The listing builds one solid part. Answer for the finished solid, in the listing's coordinates (mm). A direction names the side the tool comes from. Coordinates: 2 decimals unless noted, no trailing zeros. Write each loop counter-clockwise with the first axis right and the second up, starting at its lowest first coordinate (ties: lowest second). Pieces come first, ordered by that corner, then holes.
from build123d import *

# Parameters (mm, degrees)
F0_R     = 14.75
F1_DEPTH = 5
F2_R     = 5.25
F2_R_2   = 2.75
F3_DEPTH = 5
F4_R     = 0.5


with BuildPart() as f1:
    # F0 (on Top) → F1 (new body)
    with BuildSketch(Plane.XY):
        Circle(F0_R)
    extrude(amount=F1_DEPTH)

    # F2 (on face) → F3 (join)
    with BuildSketch(Plane.XY.offset(5)):
        Circle(F2_R)
        Circle(F2_R_2, mode=Mode.SUBTRACT)
    extrude(amount=F3_DEPTH)

    # F4
    f4_edges = [f1.edges().sort_by_distance(p)[0] for p in [
        (-14.75, 0, 0),
        (-2.75, 0, 10),
    ]]
    fillet(f4_edges, radius=F4_R)


solid = f1.part
Q1. Determine the mould class of faces 3 (the face through (0, 0, 5)), 4 (the face through (-0.1, -3.4, 10)), 5 (the face through (5, 1.6, 7.5)) for opening direction X: released by +X, released by -X, zero draft, split by the parting line, or undercut.
Answers below:
face 3: undercut
face 4: zero draft
face 5: split by the parting line
Q2. Given pin 1 (3 mm diameter, centred on x = 7, z = 4.5, fed in from -Y); pin 2 (1.5 mm diameter, centred on y = 0, z = 7, fed in from +X); pin 3 (2 mm diameter, centred on y = 6.5, z = 4.5, fed in from -X); pin 4 (6 mm diameter, centred on x = 0.5, y = -1, fed in from +Z), each flat-ended and moving along its own axis, determine where each tip first touches the part or whether it passes through.
Answers below:
pin 1: stops at y = -13.69
pin 2: stops at x = 5.25
pin 3: stops at x = -13.69
pin 4: stops at z = 10
Q3. Find the intervals of material crossed by probe 1 along Y at (x, z) = (0, 7.6); probe 2 along X at (y, z) = (-0.5, 3.5); probe 3 along Z at (x, y) = (7, 10.25), in increasing order.
Answers below:
probe 1: y = -5.25 to -2.75, 2.75 to 5.25
probe 2: x = -14.74 to 14.74
probe 3: z = 0 to 5
Q4. The part is cut by section C-C, the plane z = 2.25. Write down the section's boundary in (x, y).
Answers below:
outline: circle Ø29.5 at (0, 0)
Q5. The part is cut by section A-A, the plane y = 0. Write down the section's boundary in (x, z), then the cut area to 3 significant figures.
Answers below:
outline: (-14.75, 0.5) arc R0.5 ccw to (-14.25, 0) - (14.25, 0) arc R0.5 ccw to (14.75, 0.5) - (14.75, 5) - (5.25, 5) - (5.25, 10) - (3.25, 10) arc R0.5 ccw to (2.75, 9.5) - (2.75, 5) - (-2.75, 5) - (-2.75, 9.5) arc R0.5 ccw to (-3.25, 10) - (-5.25, 10) - (-5.25, 5) - (-14.75, 5) - close
area: 172 mm2
Q6. Which of the six approach directions +Z, -Z, +X, -X, +Y, -Y give full straight-line access (tool end or side, diameter ignored) to faces 1 (the face through (0, -6, 5)), 2 (the face through (0, 0, 0))?
Answers below:
face 1: +Z
face 2: -Z, +X, -X, +Y, -Y
